Source: CAD feature listing. Evaluate the final solid. Frame: model axes, mm. Coordinates: 2 decimals unless noted, no trailing zeros. Loops run counter-clockwise (first coordinate to the right, second up) from the corner with the lowest first, then second, coordinate; pieces in that order, holes last. Notation, with made-up numbers: (64.25, 21.25) - (99.25, 21.25) arc R17 ccw to (99.25, 36.25) - close; hole circle Ø5 at (35.25, 37.5). An arc over 180 degrees is marked (long way). Write item = value, one per line. Start each with the question number.
from build123d import *

# Parameters (mm, degrees)
CROQUIS_BASE_R          = 1.45
SALIENTE_EXTRUIR1_DEPTH = 6
REDONDEO1_R             = 1
REDONDEO2_R             = 8


with BuildPart() as part:
    # Croquis base → Saliente-Extruir1 (new body)
    with BuildSketch(Plane(origin=(0, 0, 0), x_dir=(1, 0, 0), z_dir=(0, 1, 0))):
        with BuildLine():
            Line((2.984067851, -3), (-10.738, -3))
            Line((-10.738, -3), (-12.5, -4.5))
            Line((-12.5, -4.5), (-12.6, -4.5))
            Line((-12.6, -4.5), (-12.8, -4.5))
            Line((-12.8, -4.5), (-13.15, -3.5))
            Line((-13.15, -3.5), (-13.5, -4.5))
            Line((-13.5, -4.5), (-13.7, -4.5))
            Line((-13.7, -4.5), (-14.05, -3.5))
            Line((-14.05, -3.5), (-14.4, -4.5))
            Line((-14.4, -4.5), (-14.6, -4.5))
            Line((-14.6, -4.5), (-14.95, -3.5))
            Line((-14.95, -3.5), (-15.3, -4.5))
            Line((-15.3, -4.5), (-15.5, -4.5))
            Line((-15.5, -4.5), (-15.85, -3.5))
            Line((-15.85, -3.5), (-16.2, -4.5))
            Line((-16.2, -4.5), (-16.4, -4.5))
            Line((-16.4, -4.5), (-16.75, -3.5))
            Line((-16.75, -3.5), (-17.1, -4.5))
            Line((-17.1, -4.5), (-17.3, -4.5))
            Line((-17.3, -4.5), (-17.65, -3.5))
            Line((-17.65, -3.5), (-18, -4.5))
            Line((-18, -4.5), (-18.2, -4.5))
            Line((-18.2, -4.5), (-18.55, -3.5))
            Line((-18.55, -3.5), (-18.9, -4.5))
            Line((-18.9, -4.5), (-19.1, -4.5))
            Line((-19.1, -4.5), (-19.45, -3.5))
            Line((-19.45, -3.5), (-19.8, -4.5))
            Line((-19.8, -4.5), (-20, -4.5))
            Line((-20, -4.5), (-20.35, -3.5))
            Line((-20.35, -3.5), (-20.7, -4.5))
            Line((-20.7, -4.5), (-20.9, -4.5))
            Line((-20.9, -4.5), (-21.25, -3.5))
            Line((-21.25, -3.5), (-21.6, -4.5))
            Line((-21.6, -4.5), (-21.8, -4.5))
            Line((-21.8, -4.5), (-22.15, -3.5))
            Line((-22.15, -3.5), (-22.5, -4.5))
            Line((-22.5, -4.5), (-22.7, -4.5))
            Line((-22.7, -4.5), (-23.05, -3.5))
            Line((-23.05, -3.5), (-23.4, -4.5))
            Line((-23.4, -4.5), (-23.6, -4.5))
            Line((-23.6, -4.5), (-23.95, -3.5))
            Line((-23.95, -3.5), (-24.3, -4.5))
            Line((-24.3, -4.5), (-24.5, -4.5))
            Line((-24.5, -4.5), (-24.85, -3.5))
            Line((-24.85, -3.5), (-25.2, -4.5))
            Line((-25.2, -4.5), (-25.4, -4.5))
            Line((-25.4, -4.5), (-25.75, -3.5))
            Line((-25.75, -3.5), (-26.1, -4.5))
            Line((-26.1, -4.5), (-26.3, -4.5))
            Line((-26.3, -4.5), (-26.65, -3.5))
            Line((-26.65, -3.5), (-27, -4.5))
            Line((-27, -4.5), (-27.2, -4.5))
            Line((-27.2, -4.5), (-27.55, -3.5))
            Line((-27.55, -3.5), (-27.9, -4.5))
            Line((-27.9, -4.5), (-28.1, -4.5))
            Line((-28.1, -4.5), (-28.45, -3.5))
            Line((-28.45, -3.5), (-28.8, -4.5))
            Line((-28.8, -4.5), (-29, -4.5))
            Line((-29, -4.5), (-29.35, -3.5))
            Line((-29.35, -3.5), (-29.7, -4.5))
            Line((-29.7, -4.5), (-29.9, -4.5))
            Line((-29.9, -4.5), (-30.25, -3.5))
            Line((-30.25, -3.5), (-30.6, -4.5))
            Line((-30.6, -4.5), (-30.8, -4.5))
            Line((-30.8, -4.5), (-31.15, -3.5))
            Line((-31.15, -3.5), (-31.5, -4.5))
            Line((-31.5, -4.5), (-32.5, -4.5))
            Line((-32.5, -4.5), (-32.5, -3))
            Line((-32.5, -3), (-32.5, 0.5))
            Line((-32.5, 0.5), (-30, 3))
            Line((-30, 3), (-2.984067851, 3))
            Line((-2.984067851, 3), (16.262914155, 12.309249498))
            ThreePointArc((16.262914155, 12.309249498), (21.605496986, 10.45), (19.746247488, 5.107417169))
            Line((19.746247488, 5.107417169), (2.984067851, -3))
        make_face()
        with Locations(Location((-27, -0.750184615, 0), (0, 0, 270))):
            Circle(CROQUIS_BASE_R, mode=Mode.SUBTRACT)
        with Locations(Location((0, 0, 0), (0, 0, 270))):
            Circle(CROQUIS_BASE_R, mode=Mode.SUBTRACT)
        with Locations(Location((18.004580821, 8.708333333, 0), (0, 0, 270))):
            Circle(CROQUIS_BASE_R, mode=Mode.SUBTRACT)
    extrude(amount=SALIENTE_EXTRUIR1_DEPTH)

    # Redondeo1
    redondeo1_edges = [part.edges().sort_by_distance(p)[0] for p in [
        (-30, 3, -3),
        (-32.5, 3, -0.5),
        (-32.5, 3, 4.5),
    ]]
    fillet(redondeo1_edges, radius=REDONDEO1_R - 0.0001)  # a hair under: the kernel refuses the full size

    # Redondeo2
    redondeo2_edges = [part.edges().sort_by_distance(p)[0] for p in [
        (2.984067851, 3, 3),
        (-2.984067851, 3, -3),
    ]]
    fillet(redondeo2_edges, radius=REDONDEO2_R)


solid = part.part
Item 1: Draft query along X for faces 1 (the cylindrical face through (21.566, 2.958, -10.529)), 2 (the flat face through (-25.57, 2.96, 4.01)), 3 (the flat face through (-28.62, 2.96, 3.99)), 4 (the cylindrical face through (-3.055, 3.042, -3.196)). Return one class per face: released by +X, released by -X, zero draft, split by the parting line, or undercut.
Item 2: Material intervals for L1, parallel to X at y = 0.55, z = -0.5; L2, parallel to X at y = 0.45, z = -8.25; L3, parallel to Z at x = -23.5, y = 5.25, sorted ascending. Write a range as [from, to].
Item 3: Cut plane B-B (y = 4.2). State how many separate pieces and enclosed holes the cut face has, then the cut area to 3 significant figures.
Item 4: First-contact query: pin 1 (1.8 mm diameter, centred on x = -6.5, y = 2, fed in from +Z); pin 2 (1 mm diameter, centred on y = 2, z = -6.5, fed in from +X). Flat tips, straight axial feed; report the tip coordinate or a pass-through.
Item 5: Cut plane C-C (x = -8.5). Return the cut outline in (y, z).
Item 6: Cut plane A-A (x = 0). Return the cut outline in (y, z).
Responses:
q1.face_1 = split by the parting line
q1.face_2 = undercut
q1.face_3 = undercut
q1.face_4 = released by -X
q2.L1 = [-32.41, -27.73], [-26.27, -1.36], [1.36, 10.22]
q2.L2 = [7.87, 16.63], [19.38, 21.98]
q2.L3 = [-3, 4.5]
q3.separate_pieces = 1
q3.enclosed_holes = 3
q3.area = 381 mm2
q4.pin_1 = 3
q4.pin_2 = 21.62
q5.outline = (0, -3) - (6, -3) - (6, 3) - (0, 3) - close
q6.outline = (0, -4.44) - (6, -4.44) - (6, -1.45) - (0, -1.45) - close; (0, 1.45) - (6, 1.45) - (6, 3) - (0, 3) - close
